from build123d import *

# Parameters (mm, degrees)
BOSS_EXTRUDE1_DEPTH            = 12
BOSS_EXTRUDE2_DEPTH            = 5
BOSS_EXTRUDE3_DEPTH            = 5
BOSS_EXTRUDE4_START            = 9
SKETCH4_R                      = 9.8
BOSS_EXTRUDE4_DEPTH            = 9
CUT_THICKEN1_START             = -12.3
CUT_THICKEN1_DEPTH             = 24.6
SKETCH5_W                      = 8
SKETCH5_H                      = 18
F_5_5_5_5_DIAMETER_HOLE1_D     = 5.5
F_5_5_5_5_DIAMETER_HOLE1_DEPTH = 1.5
F_5_5_5_5_DIAMETER_HOLE2_D     = 5.5


# Read off the part's stored shape, not the designer's step: Cut-Thicken1
with BuildPart() as part:
    # Sketch1 → Boss-Extrude1 (new body)
    with BuildSketch(Plane(origin=(0, 0, -11), x_dir=(-1, 0, 0), z_dir=(0, 0, -1))):
        with BuildLine():
            Line((24.25, -7.93583644), (24.25, -8.8))
            Line((24.25, -8.8), (35.75, -8.8))
            Line((35.75, -8.8), (35.75, -7.93583644))
            ThreePointArc((35.75, -7.93583644), (39.8, 0), (35.75, 7.93583644))
            Line((35.75, 7.93583644), (35.75, 8.8))
            Line((35.75, 8.8), (24.25, 8.8))
            Line((24.25, 8.8), (24.25, 7.93583644))
            ThreePointArc((24.25, 7.93583644), (20.2, 0), (24.25, -7.93583644))
        make_face()
    extrude(amount=-BOSS_EXTRUDE1_DEPTH)

    # Sketch2 → Boss-Extrude2 (add)
    with BuildSketch(Plane(origin=(0, 8.8, 0), x_dir=(-1, 0, 0), z_dir=(0, 1, 0))):
        Polygon((29.133974596, 0.5), (30.866025404, 0.5), (35.75, -2.319764048), (35.75, -7.680235952), (30.866025404, -10.5), (29.133974596, -10.5), (24.25, -7.680235952), (24.25, -2.319764048), align=None)
    extrude(amount=BOSS_EXTRUDE2_DEPTH)

    # Sketch3 → Boss-Extrude3 (add)
    with BuildSketch(Plane.XZ.offset(8.8)):
        Polygon((-35.75, -2.319764048), (-30.866025404, 0.5), (-29.133974596, 0.5), (-24.25, -2.319764048), (-24.25, -7.680235952), (-29.133974596, -10.5), (-30.866025404, -10.5), (-35.75, -7.680235952), align=None)
    extrude(amount=BOSS_EXTRUDE3_DEPTH)

    # Sketch4 → Boss-Extrude4 (add)
    with BuildSketch(Plane(origin=(0, 0, -11), x_dir=(-1, 0, 0), z_dir=(0, 0, -1)).offset(BOSS_EXTRUDE4_START)):
        with Locations((30, 0)):
            Circle(SKETCH4_R)
    extrude(amount=-BOSS_EXTRUDE4_DEPTH)

    # Cut-Thicken1 outline → Cut-Thicken1 (cut)
    with BuildSketch(Plane(origin=(0, 0, 0), x_dir=(1, 0, 0), z_dir=(0, 1, 0)).offset(CUT_THICKEN1_START)):
        Polygon((-30, 9.792007234), (-34.15, 7.396003617), (-34.15, 2.603996383), (-30, 0.207992766), (-25.85, 2.603996383), (-25.85, 7.396003617), align=None)
    extrude(amount=CUT_THICKEN1_DEPTH, mode=Mode.SUBTRACT)

    # Sketch5 → Cut-Revolve1 (revolve, cut)
    with BuildSketch(Plane(origin=(0, 0, 0), x_dir=(1, 0, 0), z_dir=(0, 1, 0))):
        with Locations((-34, 11)):
            Rectangle(SKETCH5_W, SKETCH5_H)
    revolve(axis=Axis((-30, 0, -2), (0, 0, -1)), mode=Mode.SUBTRACT)

    # Ø5.5 (5.5) Diameter Hole1
    with Locations(Plane(origin=(0, 12.3, 0), x_dir=(-1, 0, 0), z_dir=(0, -1, 0))):
        with Locations((30, 5)):
            Hole(F_5_5_5_5_DIAMETER_HOLE1_D / 2, depth=F_5_5_5_5_DIAMETER_HOLE1_DEPTH)

    # Ø5.5 (5.5) Diameter Hole2 (through all)
    with Locations(Plane(origin=(0, -12.3, 0), x_dir=(1, 0, 0), z_dir=(0, 1, 0))):
        with Locations((-30, 5)):
            Hole(F_5_5_5_5_DIAMETER_HOLE2_D / 2)


solid = part.part
For this review, take the finished solid that the model builds, in its own axes (mm). A direction names the side the tool comes from. Coordinates: 2 decimals unless noted, no trailing zeros. Order: outer loops, then holes, each group sorted by start corner. A loop starts at its lowest first (then second) coordinate and runs counter-clockwise, first axis right, second up. Notation, with made-up numbers: (78.5, 81.5) -> (127.5, 81.5) arc R11 cw to (127.5, 95.5) -> close; hole circle Ø8 at (14, 23). An arc over 180 degrees is marked (long way). Return JSON: item names as keys, results as strings.
1. Machinability: for faces 1 (the flat face through (-25.85, 10, -5)), 2 (the flat face through (-30, 11, -10.5)), 3 (the flat face through (-35.3, -8.6, -11)), which of the approach directions +Z, -Z, +X, -X, +Y, -Y give a long, thin tool a straight path to every point of the face, cutting with its end or side? Answer none if there is none.
Answer block:
{"face 1": "none", "face 2": "+X, -X, +Y", "face 3": "-Z, -X, -Y"}
2. The part is to be moulded in two halves that separate along Z. For faces 4 (the flat face through (-35.3, 8.6, -11)), 5 (the flat face through (-29.9, -8.8, -10.8)), 6 (the flat face through (-31, -13.8, -2)), say which applies: +Z half, -Z half, draft (parallel to the pull), parting line (faces both ways), or undercut.
Answer block:
{"face 4": "-Z half", "face 5": "undercut", "face 6": "draft"}
3. We need section C-C on x = -31.5. State how many separate pieces and enclosed holes the cut face has, and give its area (3 significant figures).
Answer block:
{"separate pieces": "3", "enclosed holes": "0", "area": "107 mm²"}
4. For pin 1 Ø4 at (y, z) = (10.5, -4) entering from +X; pin 2 Ø2.5 at (y, z) = (9.5, -4) entering from -X; pin 3 Ø5 at (x, y) = (-27, 0) entering from -Z; pin 4 Ø1 at (x, z) = (-29, -5) entering from +Y, all flat-tipped, find the tip position at first contact; note any pin that passes through.
Answer block:
{"pin 1": "x = -24.25", "pin 2": "x = -35.75", "pin 3": "z = -2", "pin 4": "through"}
5. For line 1 (X direction, y = 10, z = -5); line 2 (Z direction, x = -30, y = -13.2); line 3 (Y direction, x = -33, z = -7.75), list the stretches that pass through material, from the lowest coordinate up. Write a range as from..to.
Answer block:
{"line 1": "-35.75..-34.15, -25.85..-24.25", "line 2": "-10.5..-7.75, -2.25..0.5", "line 3": "-13.8..-12.3, 12.3..13.8"}
6. We need section B-B on y = -11. Write out the cut boundary in (x, z), and give its area (3 significant figures).
Answer block:
{"outline": "(-35.75, -7.68) -> (-30.87, -10.5) -> (-29.13, -10.5) -> (-24.25, -7.68) -> (-24.25, -2.32) -> (-29.13, 0.5) -> (-30.87, 0.5) -> (-35.75, -2.32) -> close; hole (-34.15, -7.4) -> (-30, -9.79) -> (-25.85, -7.4) -> (-25.85, -2.6) -> (-30, -0.21) -> (-34.15, -2.6) -> close", "area": "39.3 mm²"}
7. We need section A-A on z = -5. Write out the cut boundary in (x, y), and give its area (3 significant figures).
Answer block:
{"outline": "(-35.75, -13.8) -> (-32.75, -13.8) -> (-32.75, -12.3) -> (-34.15, -12.3) -> (-34.15, -6.84) arc R8 cw to (-34.15, 6.84) -> (-34.15, 12.3) -> (-32.75, 12.3) -> (-32.75, 13.8) -> (-35.75, 13.8) -> (-35.75, 7.94) arc R9.8 ccw to (-35.75, -7.94) -> close; (-27.25, -13.8) -> (-24.25, -13.8) -> (-24.25, -7.94) arc R9.8 ccw to (-24.25, 7.94) -> (-24.25, 13.8) -> (-27.25, 13.8) -> (-27.25, 12.3) -> (-25.85, 12.3) -> (-25.85, 6.84) arc R8 cw to (-25.85, -6.84) -> (-25.85, -12.3) -> (-27.25, -12.3) -> close", "area": "112 mm²"}
8. We need section D-D on y = 9.25. Write out the cut boundary in (x, z), and give its area (3 significant figures).
Answer block:
{"outline": "(-35.75, -7.68) -> (-30.87, -10.5) -> (-29.13, -10.5) -> (-24.25, -7.68) -> (-24.25, -2.32) -> (-29.13, 0.5) -> (-30.87, 0.5) -> (-35.75, -2.32) -> close; (-33.24, -20) -> (-26.76, -20) -> (-26.76, -11) -> (-33.24, -11) -> close; hole (-34.15, -7.4) -> (-30, -9.79) -> (-25.85, -7.4) -> (-25.85, -2.6) -> (-30, -0.21) -> (-34.15, -2.6) -> close", "area": "97.6 mm²"}
